Read the model definition and answer for the solid it produces. Units are mm, in the model's axes. A direction names the side the tool comes from. Coordinates: 2 decimals unless noted, no trailing zeros. Loops run counter-clockwise (first coordinate to the right, second up) from the corner with the lowest first, then second, coordinate; pieces in that order, holes last.
Autodesk Inventor part; units mm, degrees
ref_plane "YZ Plane" through (0, 0, 0) normal (1, 0, 0) x (0, 1, 0)
ref_plane "XZ Plane" through (0, 0, 0) normal (0, 1, 0) x (-1, 0, 0)
ref_plane "XY Plane" through (0, 0, 0) normal (0, 0, 1) x (1, 0, 0)
sketch "Sketch1" plane through (0, 0, 0) normal (0, 0, 1) x (1, 0, 0)
  line L0 (762, 0) -> (762, -101.6)
  line L1 (762, -101.6) -> (0, -101.6)
  line L2 (0, -101.6) -> (0, 0)
  line L3 (194.457, 486.6085) -> (233.372, 453.9549)
  line L4 (233.372, 453.9549) -> (102.7576, 298.2946)
  line L5 (102.7576, 298.2946) -> (63.8425, 330.9483)
  line L6 (63.8425, 330.9483) -> (194.457, 486.6085)
  line L7 (-316.8542, 110.7002) -> (-152.9915, 230.8635)
  line L8 (-152.9915, 230.8635) -> (-122.9506, 189.8979)
  line L9 (-122.9506, 189.8979) -> (-286.8134, 69.7345)
  line L10 (-286.8134, 69.7345) -> (-316.8542, 110.7002)
  circle A0 centre (97.7035, 16.2291) radius 358.4366 construction
  line L11 (-240.3853, 135.2786) -> (97.7035, 16.2291) construction
  line L12 (97.7035, 16.2291) -> (132.2805, 372.994) construction
  circle A1 centre (144.0057, 50.3583) radius 362.156 construction
  line L13 (144.0057, 50.3583) -> (164.9341, 411.9091) construction
  line L14 (144.0057, 50.3583) -> (-199.4196, 165.3194) construction
  circle A2 centre (-240.3853, 135.2786) radius 12.7
  circle A3 centre (-199.4196, 165.3194) radius 12.7
  circle A4 centre (132.2805, 372.994) radius 12.7
  circle A5 centre (164.9341, 411.9091) radius 12.7
  circle A6 centre (97.7035, 16.2291) radius 12.7
  circle A7 centre (144.0057, 50.3583) radius 12.7
  line L15 (-199.4196, 165.3194) -> (144.0057, 50.3583) construction
  arc A8 (-215.4061, 202.6622) -> (-230.8062, 191.1057) centre (-199.4196, 165.3194) ccw
  arc A9 (131.5057, 48.1134) -> (132.3942, 55.5025) centre (144.0057, 50.3583) ccw
  line L16 (-240.3853, 135.2786) -> (97.7035, 16.2291) construction
  line L17 (-244.6034, 123.2995) -> (93.4854, 4.2501)
  line L18 (101.9216, 28.2081) -> (-236.1671, 147.2576)
  arc A10 (-236.1671, 147.2576) -> (-244.6034, 123.2995) centre (-240.3853, 135.2786) ccw
  arc A11 (93.4854, 4.2501) -> (101.9216, 28.2081) centre (97.7035, 16.2291) ccw
  line L19 (164.9341, 411.9091) -> (144.0057, 50.3583) construction
  line L20 (152.2553, 412.643) -> (131.3269, 51.0922)
  line L21 (156.6845, 49.6244) -> (177.6129, 411.1752)
  arc A12 (177.6129, 411.1752) -> (152.2553, 412.643) centre (164.9341, 411.9091) ccw
  arc A13 (131.3269, 51.0922) -> (156.6845, 49.6244) centre (144.0057, 50.3583) ccw
  line L22 (132.2805, 372.994) -> (97.7035, 16.2291) construction
  line L23 (119.6397, 374.2192) -> (85.0627, 17.4542)
  line L24 (110.3443, 15.004) -> (144.9213, 371.7689)
  arc A14 (144.9213, 371.7689) -> (119.6397, 374.2192) centre (132.2805, 372.994) ccw
  arc A15 (85.0627, 17.4542) -> (110.3443, 15.004) centre (97.7035, 16.2291) ccw
  line L25 (144.0057, 50.3583) -> (-199.4196, 165.3194) construction
  line L26 (148.0371, 62.4015) -> (-195.3881, 177.3626)
  line L27 (-203.451, 153.2763) -> (139.9743, 38.3151)
  arc A16 (139.9743, 38.3151) -> (148.0371, 62.4015) centre (144.0057, 50.3583) ccw
  arc A17 (-195.3881, 177.3626) -> (-203.451, 153.2763) centre (-199.4196, 165.3194) ccw
  line L28 (162.9213, 0) -> (162.9213, 31.75)
  line L29 (61.3213, 28.575) -> (61.3213, 0)
  line L30 (162.9213, 31.75) -> (124.8213, 31.75)
  line L31 (124.8213, 38.1) -> (124.8213, 66.675)
  line L32 (127.9963, 69.85) -> (159.7463, 69.85)
  line L33 (162.9213, 66.675) -> (162.9213, 31.75)
  arc A18 (162.9213, 66.675) -> (159.7463, 69.85) centre (159.7463, 66.675) ccw
  arc A19 (127.9963, 69.85) -> (124.8213, 66.675) centre (127.9963, 66.675) ccw
  circle A20 centre (144.0057, 50.3583) radius 14.2875
  circle A21 centre (97.7035, 16.2291) radius 14.2875
  line L34 (61.3213, 0) -> (61.3213, -6.35)
  line L35 (61.3213, -6.35) -> (162.9213, -6.35)
  line L36 (162.9213, -6.35) -> (162.9213, 0)
  line L37 (124.8213, 34.925) -> (121.541, 34.925)
  line L38 (121.6463, 34.925) -> (64.4963, 34.925)
  line L39 (61.3213, 31.75) -> (61.3213, 28.575)
  arc A22 (64.4963, 34.925) -> (61.3213, 31.75) centre (64.4963, 31.75) ccw
  arc A23 (121.6463, 34.925) -> (124.8213, 38.1) centre (121.6463, 38.1) ccw
  line L40 (61.3213, -6.35) -> (61.3213, -19.05)
  line L41 (61.3213, -19.05) -> (162.9213, -19.05)
  line L42 (162.9213, -19.05) -> (162.9213, -6.35)
  line L43 (61.3213, -15.875) -> (162.9213, -15.875)
  point P0 (213.9145, 470.2817)
  point P1 (83.3001, 314.6214)
  point P2 (-301.8338, 90.2173)
  point P3 (-27.7069, 107.8389)
  point P4 (-71.3409, 75.7538)
  point P5 (154.4699, 231.1337)
  point P6 (114.992, 194.6116)
  point P7 (-27.7069, 107.8389)
  point P8 (124.8213, 69.85)
  point P9 (162.9213, 69.85)
  point P10 (132.4127, 69.85)
  point P11 (132.2867, 67.6739)
  point P12 (141.8302, 64.4792)
  point P13 (131.7052, 57.6267)
  point P14 (126.6629, 69.5564)
  point P15 (61.3213, 34.925)
  point P16 (124.8213, 43.3876)
  point P17 (157.8552, 69.85)
  point P18 (157.0627, 56.1589)
  point P19 (133.7674, 40.3929)
  point P20 (86.6269, 33.5938)
  point P21 (82.8464, 34.925)
  point P22 (86.756, 34.925)
  dimension "d0" = 762
  dimension "d1" = 101.6
  dimension "d2" = 50.8
  dimension "d3" = 203.2
  dimension "d6" = 203.2
  dimension "d7" = 50.8
  dimension "d12" = 25.4
  dimension "d13" = 25.4
  dimension "d14" = 25.4
  dimension "d15" = 25.4
  dimension "d16" = 25.4
  dimension "d17" = 25.4
  dimension "d18" = 25.4
  dimension "d19" = 25.4
  dimension "d20" = 76.2
  dimension "d21" = 76.2
  dimension "d22" = 76.2
  dimension "d23" = 76.2
  dimension "d24" = 25.4
  dimension "d25" = 25.4
  dimension "d26" = 25.4
  dimension "d27" = 25.4
  dimension "d28" = 25.4
  dimension "d29" = 25.4
  dimension "d30" = 25.4
  dimension "d32" = 31.75
  dimension "d33" = 38.1
  dimension "d34" = 38.1
  dimension "d35" = 3.175
  dimension "d43" = 28.575
  dimension "d44" = 28.575
  dimension "d45" = 6.35
  dimension "d47" = 3.175
  dimension "d65" = 12.7
  dimension "d66" = 3.175
extrude "Extrusion1" add sketch "Sketch1" along normal blind 3.175 contours L32 A18 L33 L28 L36 L35 L34 L29 L17 A21 L24 L38 L37 A23 L31 L27 A20 L21 | L21 A20 L26 L20 L32 | L20 L26 A19 L32 | L26 A20 L20 | L20 A20 L27 L31 A19 L26 | L38 L24 A21 L18 L23 | L23 L18 L38 | L23 A21 L17 L29 L39 A22 L38 L18 | L18 A21 L23 | L42 L43 L40 L35 | L42 L41 L40 L43
sketch "Sketch7" plane through (0, 0, 0) normal (0, 0, -1) x (-1, 0, 0)
  line L0 (-162.9213, -19.05) -> (-162.9213, 66.675)
  line L1 (-61.3213, -19.05) -> (-162.9213, -19.05)
  line L2 (-61.3213, 31.75) -> (-61.3213, -19.05)
  line L3 (-162.9213, -15.875) -> (-61.3213, -15.875)
  point P0 (0, 0)
  dimension "d82" = 3.175
extrude "Extrusion7" add sketch "Sketch7" along normal blind 38.1
fillet "Fillet3" radius 3.175 4 edges at (61.3213, -17.4625, -38.1) (162.9213, -17.4625, -38.1) (112.1213, -15.875, 0) (112.1213, -19.05, 3.175)
sketch "Sketch8" plane through (61.3213, -15.875, -3.175) normal (0, 1, 0) x (1, 0, 0)
  line L0 (101.6, 0) -> (101.6, 31.75)
  arc A0 (101.6, 31.75) -> (98.425, 34.925) centre (98.425, 31.75) ccw
  line L1 (3.175, 34.925) -> (98.425, 34.925)
  line L2 (0, 0) -> (0, 31.75)
  arc A1 (3.175, 34.925) -> (0, 31.75) centre (3.175, 31.75) ccw
  line L3 (101.6, 22.225) -> (0, 22.225)
  line L4 (0, 31.75) -> (0, -3.175)
  circle A2 centre (88.9, 22.225) radius 3.175
  circle A3 centre (63.5, 22.225) radius 3.175
  circle A4 centre (38.1, 22.225) radius 3.175
  circle A5 centre (12.7, 22.225) radius 3.175
  point P0 (-61.3213, -3.175)
  dimension "d86" = 12.7
  dimension "d87" = 6.35
  dimension "d88" = 6.35
  dimension "d89" = 6.35
  dimension "d90" = 6.35
  dimension "d91" = 12.7
  dimension "d92" = 25.4
  dimension "d93" = 25.4
  dimension "d94" = 25.4
extrude "Extrusion8" cut sketch "Sketch8" against normal blind 38.1 contours A2 L3 | L3 A2 | A3 L3 | L3 A3 | A4 L3 | L3 A4 | A5 L3 | L3 A5
properties part number "4-bar intake mount(alt)"
Item 1: Find the intervals of material crossed by line 1 along Z through (x, y) = (144, 19) (3 decimals); line 2 along Y through (x, z) = (151.5, -21.5) (3 decimals); line 3 along Y through (x, z) = (83, 0.5) (3 decimals), in increasing order.
Numbers:
line 1: z = 0 to 3.175
line 2: y = -19.05 to -15.875
line 3: y = -19.01 to 34.925
Item 2: Given pin 1 (1 mm diameter, centred on x = 128.5, z = -31.5, fed in from +Y) (3 decimals); pin 2 (4 mm diameter, centred on x = 74.02, z = -25.4, fed in from +Y); pin 3 (1.6 mm diameter, centred on y = 59.5, z = 2, fed in from -X); pin 4 (25 mm diameter, centred on x = 115, y = 35.5, fed in from -Z), each flat-ended and moving along its own axis, determine where each tip first touches the part or whether it passes through.
Numbers:
pin 1: stops at y = -15.875
pin 2: passes through
pin 3: stops at x = 124.82
pin 4: stops at z = 0
Item 3: A cutting plane is placed at C-C on y = 20. Determine the outline of the cut face in (x, z) (3 decimals).
Numbers:
outline: (61.321, 0) - (83.923, 0) - (83.923, 3.175) - (61.321, 3.175) - close; (111.484, 0) - (162.921, 0) - (162.921, 3.175) - (111.484, 3.175) - close
Item 4: A cutting plane is placed at B-B on x = 135. Determine the outline of the cut face in (y, z) (3 decimals), then the cut area to 3 significant figures.
Numbers:
outline: (-19.05, -38.1) - (-15.875, -38.1) - (-15.875, -3.175) arc R3.175 cw to (-12.7, 0) - (39.266, 0) - (39.266, 3.175) - (-15.875, 3.175) arc R3.175 ccw to (-19.05, 0) - close; (61.45, 0) - (69.85, 0) - (69.85, 3.175) - (61.45, 3.175) - close
area: 333 mm2
Item 5: Determine the mould class of faces 1 (the face through (149.81, -17.44, -28.55)), 2 (the face through (113, -15.875, -20)), 3 (the face through (62.23, -17.48, -37.15)) for opening direction X: released by +X, released by -X, zero draft, split by the parting line, or undercut.
Numbers:
face 1: undercut
face 2: zero draft
face 3: released by -X
Item 6: A cutting plane is placed at D-D on y = 40.5. Determine the outline of the cut face in (x, z) (3 decimals).
Numbers:
outline: (124.821, 0) - (133.664, 0) - (133.664, 3.175) - (124.821, 3.175) - close; (154.347, 0) - (162.921, 0) - (162.921, 3.175) - (154.347, 3.175) - close
Item 7: Which of the six approach directions +Z, -Z, +X, -X, +Y, -Y give full straight-line access (tool end or side, diameter ignored) to faces 4 (the face through (162.921, 11, 1)), 5 (the face through (111.4, 10.8, 0)), 6 (the face through (93, 34.925, 2))?
Numbers:
face 4: +Z, -Z, +X, +Y, -Y
face 5: -Z, +X, -X, +Y
face 6: +Z, -Z, -X, +Y
Item 8: A cutting plane is placed at A-A on z = -25.4. Determine the outline of the cut face in (x, y) (3 decimals).
Numbers:
outline: (61.321, -19.05) - (70.846, -19.05) - (70.846, -15.875) - (61.321, -15.875) - close; (77.196, -19.05) - (96.246, -19.05) - (96.246, -15.875) - (77.196, -15.875) - close; (102.596, -19.05) - (121.646, -19.05) - (121.646, -15.875) - (102.596, -15.875) - close; (127.996, -19.05) - (147.046, -19.05) - (147.046, -15.875) - (127.996, -15.875) - close; (153.396, -19.05) - (162.921, -19.05) - (162.921, -15.875) - (153.396, -15.875) - close
